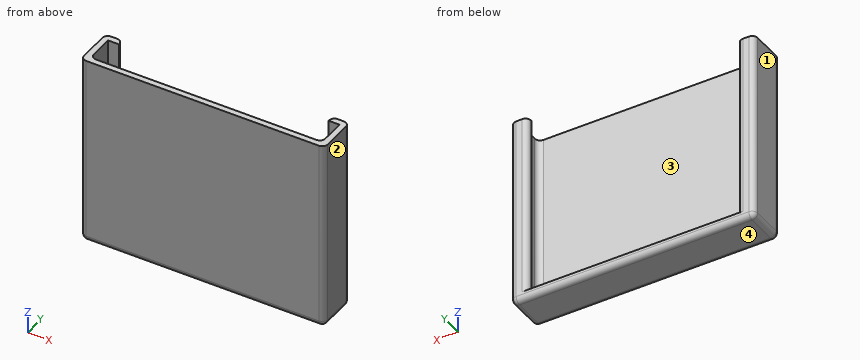
```python
from build123d import *

# Parameters (mm, degrees)
F1_DEPTH = 70
F3_DEPTH = 3
F4_R     = 2


with BuildPart() as f1:
    # F0 (on Top) → F1 (new body)
    with BuildSketch(Plane.XY):
        Polygon((-44.45, 0), (0, 0), (0, 2.2), (-42.25, 2.2), (-42.25, 12.7), (-38.25, 12.7), (-38.25, 14.9), (-44.45, 14.9), align=None)
        Polygon((0, 2.2), (0, 0), (44.45, 0), (44.45, 14.6), (44.45, 14.9), (38.25, 14.9), (38.25, 12.7), (42.25, 12.7), (42.25, 2.2), align=None)
    extrude(amount=F1_DEPTH)

    # F2 (on face) → F3 (join)
    with BuildSketch(Plane.XY):
        Polygon((0, 0), (44.45, 0), (44.45, 14.9), (-38.25, 14.9), (-38.25, 12.7), (-42.25, 12.7), (-42.25, 2.2), (0, 2.2), align=None)
        Polygon((-44.45, 0), (0, 0), (0, 2.2), (-42.25, 2.2), (-42.25, 12.7), (-38.25, 12.7), (-38.25, 14.9), (-44.45, 14.9), align=None)
    extrude(amount=F3_DEPTH)

    # F4
    f4_edges = [f1.edges().sort_by_distance(p)[0] for p in [
        (44.45, 0, 35),
        (44.45, 14.9, 35),
        (38.25, 14.9, 36.5),
        (42.25, 2.2, 36.5),
        (-38.25, 14.9, 36.5),
        (-42.25, 2.2, 36.5),
        (-44.45, 14.9, 35),
        (-44.45, 0, 35),
        (0, 0, 0),
        (0, 14.9, 0),
        (-44.45, 7.45, 0),
        (44.45, 7.45, 0),
    ]]
    fillet(f4_edges, radius=F4_R)


solid = f1.part
```
Model file for the job. Use its own axes, mm. Face numbers are marked on the shaded views. Coordinates: 2 decimals unless noted, no trailing zeros. Loops run counter-clockwise (first coordinate to the right, second up) from the corner with the lowest first, then second, coordinate; pieces in that order, holes last. Notation, with made-up numbers: M 68.25,-14 L 118.25,-14 A17 ccw 118.25,10 Z; hole C 68,80 d9. An arc over 180 degrees is marked long. Use CSV: the item, a comma, the result in double quotes. Start each with the question number.
1. Two-plate mould, pull along X, no slides. Class the marked faces 1, 2, 3 and 4: pulls with the +X half, pulls with the -X half, needs draft (parallel to the pull), parting line crosses it, or undercut.
2. Band-saw the part on B-B, the plane x = -24. List the corners of the cut face in (y, z).
3. Flat gauge pin, fed straight in: pin 1 (8 mm diameter, centred on x = 25.5, y = 12.5, fed in from +Z). Where does the tip first touch, or does it go through?
4. Band-saw the part on C-C, the plane y = 9. List the corners of the cut face in (x, z).
5. Band-saw the part on A-A, the plane z = 35.5. List the corners of the cut face in (x, y), then the cut area to 3 significant figures.
6. Probe probe 1 along X at (y, z) = (6, 27); probe 2 along X at (y, z) = (13, 21.5); probe 3 along Z at (x, y) = (-35, 11.75). List the from-to ranges inside material, lowest first. Write a range as [from, to].
Entries:
1,face 1,"pulls with the -X half"
1,face 2,"pulls with the +X half"
1,face 3,"undercut"
1,face 4,"needs draft"
2,outline,"M 0,2 A2 ccw 2,0 L 12.9,0 A2 ccw 14.9,2 L 14.9,3 L 2.2,3 L 2.2,70 L 0,70 Z"
3,pin 1,"stops at z = 3"
4,outline,"M -44.45,2 A2 ccw -42.45,0 L 42.45,0 A2 ccw 44.45,2 L 44.45,70 L 42.25,70 L 42.25,3 L -42.25,3 L -42.25,70 L -44.45,70 Z"
5,outline,"M -44.45,2 A2 ccw -42.45,0 L 42.45,0 A2 ccw 44.45,2 L 44.45,12.9 A2 ccw 42.45,14.9 L 40.25,14.9 A2 ccw 38.25,12.9 L 38.25,12.7 L 42.25,12.7 L 42.25,4.2 A2 cw 40.25,2.2 L -40.25,2.2 A2 cw -42.25,4.2 L -42.25,12.7 L -38.25,12.7 L -38.25,12.9 A2 ccw -40.25,14.9 L -42.45,14.9 A2 ccw -44.45,12.9 Z"
5,area,"266 mm2"
6,probe 1,"x = [-44.45, -42.25], [42.25, 44.45]"
6,probe 2,"x = [-44.45, -38.25], [38.25, 44.45]"
6,probe 3,"z = [0, 3]"
